from build123d import *
from build123d.topology import SkipClean

# Parameters (mm, degrees)
BOSS_EXTRUDE1_DEPTH                                 = 13.7795
SKETCH3_R                                           = 1.27
CUT_EXTRUDE1_DEPTH                                  = 28.24278526
BOSS_EXTRUDE3_REACH                                 = 29.243
SKETCH4_R                                           = 3.024456955
BOSS_EXTRUDE3_DIRECTION_2_REACH                     = 29.243
CUT_EXTRUDE2_START                                  = -27.686
SKETCH5_R                                           = 1.27
CUT_EXTRUDE2_DEPTH                                  = 27.686
SKETCH6_W                                           = 5.3594
SKETCH6_H                                           = 6.04891391
SKETCH6_W_2                                         = 8.5598
CUT_EXTRUDE3_DEPTH                                  = 27.163772894
FILLET1_R                                           = 2.54
BOSS_EXTRUDE5_DEPTH                                 = 2.54
SKETCH8_R                                           = 1.905
BOSS_EXTRUDE6_DEPTH                                 = 5.207
CBORE_FOR_00_BINDING_HEAD_MACHINE_SCREW_D           = 1.397
CBORE_FOR_00_BINDING_HEAD_MACHINE_SCREW_DEPTH       = 3.81
CBORE_FOR_00_BINDING_HEAD_MACHINE_SCREW_CBORE_D     = 2.54
CBORE_FOR_00_BINDING_HEAD_MACHINE_SCREW_CBORE_DEPTH = 0.889
CBORE_FOR_00_BINDING_HEAD_MACHINE_SCREW_TIP         = 0.419701142
FILLET3_R                                           = 0.635


with BuildPart() as part:
    # Sketch2 → Boss-Extrude1 (new, symmetric)
    with BuildSketch(Plane(origin=(0, 0, 0), x_dir=(0, 0, -1), z_dir=(1, 0, 0))):
        Polygon((0.358296425, 8.382), (0, 6.35), (0, 0), (2.54, 0), (2.54, 6.35), (2.898296425, 8.382), (5.451158451, 22.86), (2.911158451, 22.86), align=None)
    extrude(amount=BOSS_EXTRUDE1_DEPTH, both=True)

    # Sketch3 → Cut-Extrude1 (cut, through all)
    with BuildSketch(Plane.XY):
        with Locations((-10.8585, 3.039071392)):
            Circle(SKETCH3_R)
        with Locations((10.8585, 3.039071392)):
            Circle(SKETCH3_R)
        with BuildLine():
            Line((-6.093079, 2.794), (6.093079, 2.794))
            ThreePointArc((6.093079, 2.794), (7.395567274, 2.453324554), (8.364453302, 1.518554352))
            ThreePointArc((8.364453302, 1.518554352), (11.648161508, 0.226834613), (13.7795, 3.039071392))
            Line((13.7795, 3.039071392), (14.4145, 3.039071392))
            Line((14.4145, 3.039071392), (14.4145, -0.635))
            Line((14.4145, -0.635), (-14.4145, -0.635))
            Line((-14.4145, -0.635), (-14.4145, 3.039071392))
            Line((-14.4145, 3.039071392), (-13.7795, 3.039071392))
            ThreePointArc((-13.7795, 3.039071392), (-11.648161508, 0.226834613), (-8.364453302, 1.518554352))
            ThreePointArc((-8.364453302, 1.518554352), (-7.395567274, 2.453324554), (-6.093079, 2.794))
        make_face()
        Polygon((-14.4145, 11.43), (-8.4201, 11.43), (-8.4201, 22.86), (-4.2799, 22.86), (-4.2799, 11.43), (4.2799, 11.43), (4.2799, 22.86), (8.4201, 22.86), (8.4201, 11.43), (14.4145, 11.43), (14.4145, 23.495), (-14.4145, 23.495), align=None)
    extrude(amount=-CUT_EXTRUDE1_DEPTH, mode=Mode.SUBTRACT)

    # Boss-Extrude3: up to this face of the body (flat: up to its plane)
    boss_extrude3_end = Plane(part.part.faces().sort_by_distance((13.7795, 7.234535696, -1.541147855))[0])
    # Sketch4 → Boss-Extrude3 (add, up to the picked face)
    with BuildSketch(Plane(origin=(0, 0, 0), x_dir=(0, 0, -1), z_dir=(1, 0, 0)), mode=Mode.PRIVATE) as boss_extrude3_sk1:
        with Locations(Location((5.070856, 17.6911, 0), (0, 0, 180))):
            Circle(SKETCH4_R)
    boss_extrude3_tool1 = split(extrude(boss_extrude3_sk1.sketch, amount=BOSS_EXTRUDE3_REACH, mode=Mode.PRIVATE), bisect_by=boss_extrude3_end, keep=Keep.BOTH, mode=Mode.PRIVATE)
    add(boss_extrude3_tool1.solids().sort_by(Axis((0, 17.6911, -5.070856), (1, 0, 0)))[0])

    # Boss-Extrude3 direction 2: up to this face of the body (flat: up to its plane)
    boss_extrude3_direction_2_end = Plane(part.part.faces().sort_by_distance((-13.7795, 7.234535696, -1.541147855))[0])
    # Sketch4 → Boss-Extrude3 direction 2 (add, up to the picked face)
    with BuildSketch(Plane(origin=(0, 0, 0), x_dir=(0, 0, -1), z_dir=(1, 0, 0)), mode=Mode.PRIVATE) as boss_extrude3_direction_2_sk1:
        with Locations(Location((5.070856, 17.6911, 0), (0, 0, 180))):
            Circle(SKETCH4_R)
    boss_extrude3_direction_2_tool1 = split(extrude(boss_extrude3_direction_2_sk1.sketch, amount=-BOSS_EXTRUDE3_DIRECTION_2_REACH, mode=Mode.PRIVATE), bisect_by=boss_extrude3_direction_2_end, keep=Keep.BOTH, mode=Mode.PRIVATE)
    add(boss_extrude3_direction_2_tool1.solids().sort_by(Axis((0, 17.6911, -5.070856), (-1, 0, 0)))[0])

    # Sketch5 → Cut-Extrude2 (cut)
    with SkipClean():  # the faces are left unmerged after this step: merging them gives an invalid solid
        with BuildSketch(Plane(origin=(13.7795, 0, 0), x_dir=(0, 0, -1), z_dir=(1, 0, 0)).offset(CUT_EXTRUDE2_START)):
            with Locations((5.070856, 17.6911)):
                Circle(SKETCH5_R)
            with BuildLine():
                Line((2.092347342, 18.216291439), (2.911158451, 22.86))
                Line((2.911158451, 22.86), (5.451158451, 22.86))
                Line((5.451158451, 22.86), (5.073035146, 20.71555617))
                ThreePointArc((5.073035146, 20.71555617), (3.12760733, 20.008668658), (2.092347342, 18.216291439))
            make_face()
        extrude(amount=CUT_EXTRUDE2_DEPTH, mode=Mode.SUBTRACT)

    # Sketch6 → Cut-Extrude3 (cut, through all)
    with BuildSketch(Plane.XY):
        with Locations((-11.0998, 17.6911)):
            Rectangle(SKETCH6_W, SKETCH6_H)
        with Locations((0, 17.6911)):
            Rectangle(SKETCH6_W_2, SKETCH6_H)
        with Locations((11.0998, 17.6911)):
            Rectangle(SKETCH6_W, SKETCH6_H)
    extrude(amount=-CUT_EXTRUDE3_DEPTH, mode=Mode.SUBTRACT)

    # Fillet1
    fillet1_edges = [part.edges().sort_by_distance(p)[0] for p in [
        (-6.35, 14.848295543, -4.038478794),
        (6.35, 14.848295543, -4.038478794),
    ]]
    fillet(fillet1_edges, radius=FILLET1_R)

    # Sketch7 → Boss-Extrude5 (add)
    with BuildSketch(Plane.ZY.offset(8.4201)):
        with BuildLine():
            Line((0, 6.35), (2.54, 6.35))
            ThreePointArc((2.54, 6.35), (0.810559409, 13.256647786), (-2.636800213, 19.486291439))
            ThreePointArc((-2.636800213, 19.486291439), (-2.29107391, 18.882801056), (-2.092347342, 18.216291439))
            Line((-2.092347342, 18.216291439), (0, 6.35))
        make_face()
    boss_extrude5 = extrude(amount=-BOSS_EXTRUDE5_DEPTH)

    # Mirror1: Boss-Extrude5 across plane
    add(boss_extrude5.mirror(Plane(origin=(0, 0, 0), x_dir=(0, 0, 1), z_dir=(1, 0, 0))))

    # Sketch8 → Boss-Extrude6 (add)
    with BuildSketch(Plane(origin=(0, 0, -2.54), x_dir=(-1, 0, 0), z_dir=(0, 0, -1))):
        with Locations(Location((7.1501, 7.112, 0), (0, 0, 90))):
            Circle(SKETCH8_R)
        with Locations(Location((-7.1501, 7.112, 0), (0, 0, 90))):
            Circle(SKETCH8_R)
    extrude(amount=-BOSS_EXTRUDE6_DEPTH)

    # CBORE for #00 Binding Head Machine Screw1
    with Locations(Plane.XY.offset(2.667)):
        with Locations((-7.1501, 7.112), (7.1501, 7.112)):
            CounterBoreHole(CBORE_FOR_00_BINDING_HEAD_MACHINE_SCREW_D / 2, CBORE_FOR_00_BINDING_HEAD_MACHINE_SCREW_CBORE_D / 2, CBORE_FOR_00_BINDING_HEAD_MACHINE_SCREW_CBORE_DEPTH, depth=CBORE_FOR_00_BINDING_HEAD_MACHINE_SCREW_DEPTH)
            with Locations((0, 0, -(CBORE_FOR_00_BINDING_HEAD_MACHINE_SCREW_DEPTH + CBORE_FOR_00_BINDING_HEAD_MACHINE_SCREW_TIP / 2))):  # 118° drill point
                Cone(0, CBORE_FOR_00_BINDING_HEAD_MACHINE_SCREW_D / 2, CBORE_FOR_00_BINDING_HEAD_MACHINE_SCREW_TIP, mode=Mode.SUBTRACT)

    # Fillet3
    fillet3_edges = [part.edges().sort_by_distance(p)[0] for p in [
        (-13.7795, 11.43, -2.165741062),
        (13.7795, 11.43, -2.165741062),
        (8.4201, 11.43, -2.165741062),
        (4.2799, 11.43, -2.165741062),
        (-4.2799, 11.43, -2.165741062),
        (-8.4201, 11.43, -2.165741062),
    ]]
    fillet(fillet3_edges, radius=FILLET3_R)


solid = part.part
The listing builds one solid part. Answer for the finished solid, in the listing's coordinates (mm). A direction names the side the tool comes from. Give positions to 0.01 mm unless a question says otherwise; leave off trailing zeros. Write each loop counter-clockwise with the first axis right and the second up, starting at its lowest first coordinate (ties: lowest second). Pieces come first, ordered by that corner, then holes. Notation, with made-up numbers: (-5.5, 53.5) -> (50.5, 53.5) arc R11 ccw to (50.5, 67.5) -> close; hole circle Ø8 at (-16, 70). An arc over 180 degrees is marked (long way). One line per question, with ' | ' between items. Start each with the question number.
1. Given pin 1 Ø1.9 at (x, y) = (-5.5, 4) entering from -Z; pin 2 Ø1.5 at (x, y) = (-2, 18) entering from +Z; pin 3 Ø1.3 at (x, z) = (-2.5, -2) entering from -Y; pin 4 Ø5 at (x, y) = (5, 3) entering from +Z, each flat-ended and moving along its own axis, determine where each tip first touches the part or whether it passes through.
2. Find the intervals of material crossed by probe 1 along X at (y, z) = (12, -1.5); probe 2 along Z at (x, y) = (5.25, 18.25); probe 3 along Y at (x, z) = (-10.25, -2.5), in increasing order.
3. Section D-D (z = -6) is taken. Determine the outline of the cut face in (x, y).
4. Section C-C (y = 13.25) is taken. Determine the outline of the cut face in (x, z).
5. Section B-B (z = 0.75) is taken. Determine the outline of the cut face in (x, y) (1 decimal).
6. For faces 4 (the flat face through (4.28, 16, -5)), 5 (the cylindrical face through (-7.412, 2.444, -1.252)), 6 (the flat face through (0, 4, 0)), 7 (the cylindrical face through (-6.635, 7.584, 0.297)), determine the directions among +Z, -Z, +X, -X, +Y, -Y from which every point of the face is accessible in a straight line to the end or side of a thin tool.
7. Section A-A (x = -0.5) is taken. Determine the outline of the cut face in (y, z), plus the area to 3 significant figures.
8. For a pull along Y with two mould halves and no side action, classify faces 1 (the conical face through (-7.034, 7.148, -1.49)), 2 (the flat face through (8.42, 15, -3)), 3 (the flat face through (11, 11.43, -2)) as pulls with the +Y half, pulls with the -Y half, needs draft (parallel to the pull), parting line crosses it, or undercut.
Response values:
1) pin 1: z = -2.54 | pin 2: through | pin 3: y = 2.79 | pin 4: z = 0
2) probe 1: -8.42 to -4.28, 4.28 to 8.42 | probe 2: -8.04 to -6.21, -3.93 to -2.1 | probe 3: 0.18 to 1.92, 4.15 to 11.43
3) outline: (-8.42, 14.81) -> (-4.28, 14.81) -> (-4.28, 16.83) -> (-8.42, 16.83) -> close; (-8.42, 18.56) -> (-4.28, 18.56) -> (-4.28, 20.57) -> (-8.42, 20.57) -> close; (4.28, 14.81) -> (8.42, 14.81) -> (8.42, 16.83) -> (4.28, 16.83) -> close; (4.28, 18.56) -> (8.42, 18.56) -> (8.42, 20.57) -> (4.28, 20.57) -> close
4) outline: (-8.42, -3.83) -> (-4.28, -3.83) -> (-4.28, -1.22) -> (-5.88, -1.22) -> (-5.88, 0.81) -> (-8.42, 0.81) -> close; (4.28, -3.83) -> (8.42, -3.83) -> (8.42, 0.81) -> (5.88, 0.81) -> (5.88, -1.22) -> (4.28, -1.22) -> close
5) outline: (-8.4, 8.5) arc R1.9 ccw (long way) to (-5.9, 8.5) -> (-5.9, 13.4) -> (-8.4, 13.4) -> close; (5.9, 8.5) arc R1.9 ccw (long way) to (8.4, 8.5) -> (8.4, 13.4) -> (5.9, 13.4) -> close; hole circle Ø1.4 at (-7.2, 7.1); hole circle Ø1.4 at (7.2, 7.1)
6) face 4: +Z, -Z, +Y | face 5: +Z, -Z, -Y | face 6: +Z, -Y | face 7: +Z
7) outline: (2.79, -2.54) -> (6.35, -2.54) -> (11.43, -3.44) -> (11.43, -0.9) -> (6.35, 0) -> (2.79, 0) -> close | area: 21.9 mm2
8) face 1: undercut | face 2: needs draft | face 3: pulls with the +Y half
